For this review, use the dimensioned drawing (mm, ordinates from the lowest corner) and the shaded views. A direction names the side the tool comes from. Coordinates: 2 decimals unless noted, no trailing zeros. Loops run counter-clockwise (first coordinate to the right, second up) from the corner with the lowest first, then second, coordinate; pieces in that order, holes last. Notation, with made-up numbers: (38.25, 82.5) - (84.25, 82.5) arc R12 cw to (84.25, 99.5) - close; hole circle Ø10 at (45, 11). An arc over 180 degrees is marked (long way). Answer in a Markdown table with one row per item. Add a question column.
(1) For P1, Ø1.5, axis at y = 39.8, z = 11.625, coming from the +X side, flat-tipped, find the tip position at first contact; note if it passes through.
(2) We need section C-C on z = 2.75. Write out the cut boundary in (x, y).
(3) Mouldability with a two-part tool opening along X and no side actions: class the marked faces 1, 2 and 3 as +X half, -X half, draft (parallel to the pull), parting line (faces both ways), or undercut.
(4) We need section D-D on y = 39.8. Write out the cut boundary in (x, z) (3 decimals), plus the area to 4 significant figures.
(5) We need section B-B on y = 31.5. Write out the cut boundary in (x, z).
(6) For line 1 along X through (y, z) = (17.5, 6); line 2 along Y through (x, z) = (28.5, 23.25); line 3 along Z through (x, y) = (43, 6.5) (3 decimals), list the stretches that pass through material, from the lowest coordinate up.
(7) We need section A-A on x = 3. Write out the cut boundary in (y, z).
(8) Machinability: for the marked faces 4 and 5, which of the approach directions +Z, -Z, +X, -X, +Y, -Y give a long, thin tool a straight path to every point of the face, cutting with its end or side? Answer none if there is none.
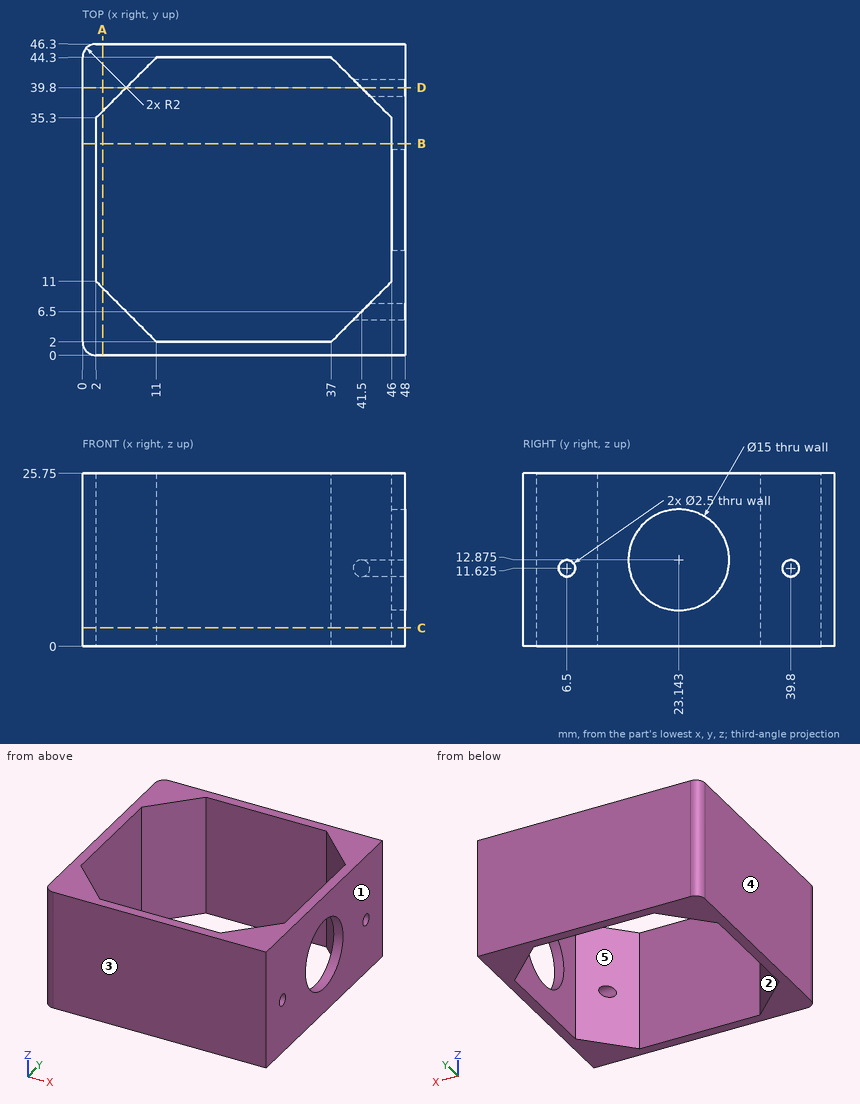
Outcome:
| question | item | result |
|---|---|---|
| 1 | P1 | x = 7.25 |
| 2 | outline | (0, 2) arc R2 ccw to (2, 0) - (48, 0) - (48, 46.3) - (2, 46.3) arc R2 ccw to (0, 44.3) - close; hole (2, 11) - (11, 2) - (37, 2) - (46, 11) - (46, 35.3) - (37, 44.3) - (11, 44.3) - (2, 35.3) - close |
| 3 | face 1 | +X half |
| 3 | face 2 | undercut |
| 3 | face 3 | draft |
| 4 | outline | (0, 0) - (6.5, 0) - (6.5, 25.75) - (0, 25.75) - close; (41.5, 0) - (48, 0) - (48, 10.375) - (41.5, 10.375) - close; (41.5, 12.875) - (48, 12.875) - (48, 25.75) - (41.5, 25.75) - close |
| 4 | area | 318.5 mm² |
| 5 | outline | (0, 0) - (2, 0) - (2, 25.75) - (0, 25.75) - close; (46, 0) - (48, 0) - (48, 25.75) - (46, 25.75) - close |
| 6 | line 1 | 0 to 2, 46 to 48 |
| 6 | line 2 | 0 to 2, 44.3 to 46.3 |
| 6 | line 3 | 0 to 10.375, 12.875 to 25.75 |
| 7 | outline | (0, 0) - (10, 0) - (10, 25.75) - (0, 25.75) - close; (36.3, 0) - (46.3, 0) - (46.3, 25.75) - (36.3, 25.75) - close |
| 8 | face 4 | +Z, -Z, -X, +Y, -Y |
| 8 | face 5 | +Z, -Z |
